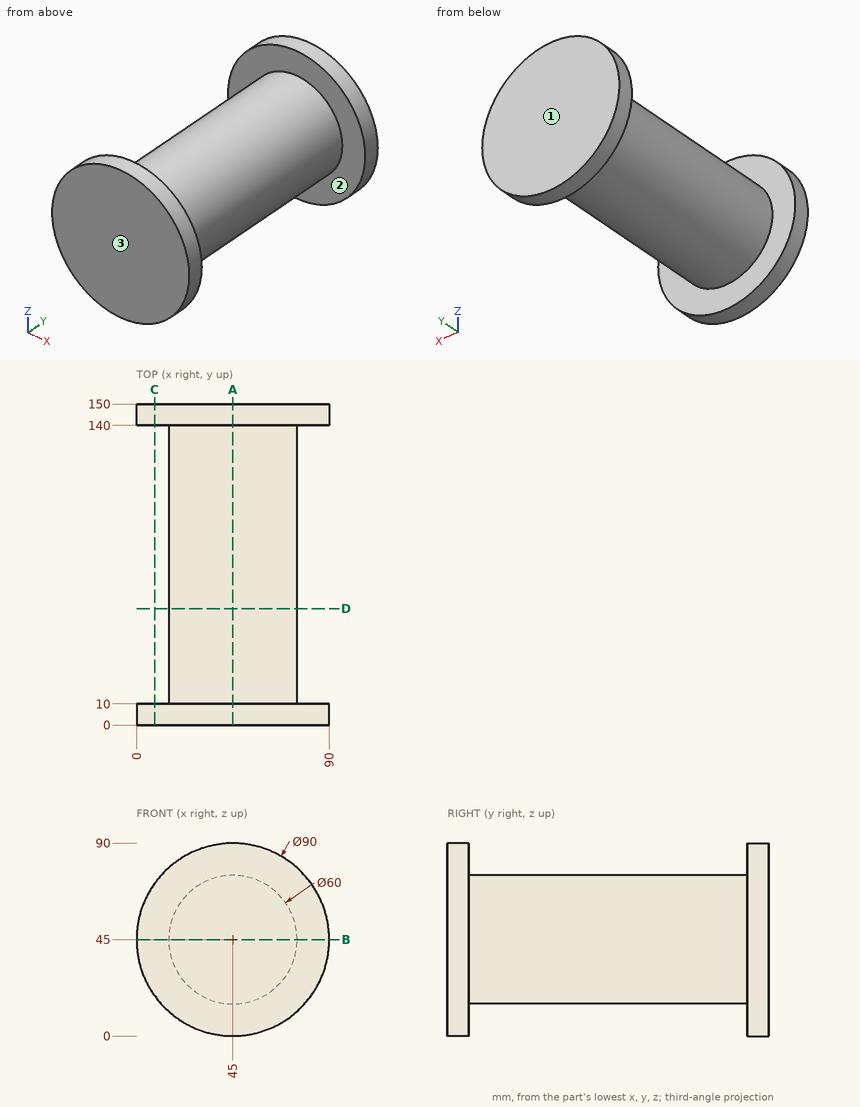
Study the drawing (mm; zero at the part's minimum x, y, z) and answer. Round coordinates to 2 decimals unless told otherwise and drop trailing zeros. Write each loop counter-clockwise with the first axis right and the second up, starting at its lowest first coordinate (ties: lowest second). Pieces come first, ordered by that corner, then holes. Notation, with made-up numbers: (88, 77.5) - (112, 77.5) arc R10 ccw to (112, 95.5) - close; hole circle Ø9 at (-0.75, 32). An arc over 180 degrees is marked (long way). Use CSV: the item, a comma, the result in double quotes.
Q1. Determine the mould class of the marked faces 1, 2 and 3 for opening direction Y: +Y half, -Y half, draft (parallel to the pull), parting line (faces both ways), or undercut.
Values:
face 1,"+Y half"
face 2,"undercut"
face 3,"-Y half"
Q2. Find section A-A, the plane x = 45. Write down the section's boundary in (y, z).
Values:
outline,"(0, 0) - (10, 0) - (10, 15) - (140, 15) - (140, 0) - (150, 0) - (150, 90) - (140, 90) - (140, 75) - (10, 75) - (10, 90) - (0, 90) - close"
Q3. Find section C-C, the plane x = 8.5. Write down the section's boundary in (y, z), then the cut area to 3 significant figures.
Values:
outline,"(0, 18.68) - (10, 18.68) - (10, 71.32) - (0, 71.32) - close; (140, 18.68) - (150, 18.68) - (150, 71.32) - (140, 71.32) - close"
area,"1,050 mm²"
Q4. Each of these flat-tipped pins is pushed along its axis until it touches: pin 1 Ø12 at (x, y) = (18.5, 47.5) entering from -Z; pin 2 Ø1 at (x, y) = (18, 27.5) entering from +Z; pin 3 Ø2 at (y, z) = (111, 36.5) entering from -X. Where does it stop, or does it pass through?
Values:
pin 1,"stops at z = 23.1"
pin 2,"stops at z = 59.06"
pin 3,"stops at x = 15.95"
Q5. Straight lines are drawn through the part: line 1 along Y through (x, z) = (57, 7); line 2 along Z through (x, y) = (46, 70.5). For each, find the intervals that lie inside material, in ascending order.
Values:
line 1,"y = 0 to 10, 140 to 150"
line 2,"z = 15.02 to 74.98"
Q6. Find section B-B, the plane z = 45. Write down the section's boundary in (x, y), then the cut area to 3 significant figures.
Values:
outline,"(0, 0) - (90, 0) - (90, 10) - (75, 10) - (75, 140) - (90, 140) - (90, 150) - (0, 150) - (0, 140) - (15, 140) - (15, 10) - (0, 10) - close"
area,"9,600 mm²"
Q7. Find section D-D, the plane y = 54.5. Write down the section's boundary in (x, z).
Values:
outline,"circle Ø60 at (45, 45)"
